Autodesk Inventor part; units mm, degrees
ref_plane "YZ Plane" through (0, 0, 0) normal (1, 0, 0) x (0, 1, 0)
ref_plane "XZ Plane" through (0, 0, 0) normal (0, 1, 0) x (-1, 0, 0)
ref_plane "XY Plane" through (0, 0, 0) normal (0, 0, 1) x (1, 0, 0)
sketch "Boceto1" plane through (0, 0, 0) normal (0, 1, 0) x (-1, 0, 0)
  line L0 (-12.5, 6.5) -> (12.5, 6.5)
  line L1 (12.5, 6.5) -> (12.5, -6.5)
  line L2 (12.5, -6.5) -> (-12.5, -6.5)
  line L3 (-12.5, -6.5) -> (-12.5, 6.5)
  line L4 (-12.5, 6.5) -> (12.5, -6.5) construction
  line L5 (12.5, 6.5) -> (-12.5, -6.5) construction
  point P0 (0, 0)
  dimension "d0" = 13
  dimension "d1" = 25
extrude "Extrusión1" add sketch "Boceto1" along normal blind 1.5
sketch "Boceto2" plane through (0, 1.5, 0) normal (0, 1, 0) x (1, 0, 0)
  circle A0 centre (-3.5, 0) radius 2.75
  line L0 (-12.5, 6.5) -> (-12.5, -6.5)
  point P0 (0, 0)
  dimension "d4" = 9
  dimension "d5" = 5.5
extrude "Extrusión2" cut sketch "Boceto2" against normal blind 1.5
sketch "Boceto3" plane through (0, 1.5, 0) normal (0, 1, 0) x (1, 0, 0)
  line L0 (-9.2, -5.5) -> (2.8, -5.5)
  line L1 (2.8, -5.5) -> (2.8, 5.5)
  line L2 (2.8, 5.5) -> (-9.2, 5.5)
  line L3 (-9.2, 5.5) -> (-9.2, -5.5)
  line L4 (-12.5, 6.5) -> (-12.5, -6.5)
  line L5 (12.5, 6.5) -> (-12.5, 6.5)
  circle A0 centre (-3.5, 0) radius 2.75
  circle A1 centre (-3.5, 0) radius 2
  point P0 (0, 0)
  dimension "d8" = 11
  dimension "d9" = 12
  dimension "d10" = 3.3
  dimension "d11" = 1
  dimension "d14" = 4
extrude "Extrusión3" add sketch "Boceto3" along normal blind 2 contours L3 L2 L1 L0 | A0
chamfer "Chaflán1" distance 3 angle 45 2 edges at (-9.2, 2.5, 5.5) (-9.2, 2.5, -5.5)
sketch "Boceto4" plane through (0, 3.5, 0) normal (0, 1, 0) x (1, 0, 0)
  circle A0 centre (-3.5, 0) radius 2
  line L0 (-2.5075, -1.7363) -> (-2.5075, 1.7363)
  point P0 (0, 0)
extrude "Extrusión4" add sketch "Boceto4" against normal up to surface (2 mm away) contours A0 L0 picked at (-2.1717, 0)
properties part number "AngleSensor"
The listing builds one solid part. Answer for the finished solid, in the listing's coordinates (mm). A direction names the side the tool comes from. Coordinates: 2 decimals unless noted, no trailing zeros. Write each loop counter-clockwise with the first axis right and the second up, starting at its lowest first coordinate (ties: lowest second). Pieces come first, ordered by that corner, then holes. Notation, with made-up numbers: M 47.5,-37.75 L 84.5,-37.75 A16 cw 84.5,-17.75 Z; hole C 74,67.25 d6. An arc over 180 degrees is marked long. Use one line per item in the form item = value.
Item 1: Find section B-B, the plane z = 0. Give the vertices of the cut face in (x, y), plus the area to 3 significant figures.
Model answer:
outline = M -12.5,0 L -6.25,0 L -6.25,1.5 L -5.5,1.5 L -5.5,3.5 L -9.2,3.5 L -9.2,1.5 L -12.5,1.5 Z; M -2.51,1.5 L -0.75,1.5 L -0.75,0 L 12.5,0 L 12.5,1.5 L 2.8,1.5 L 2.8,3.5 L -2.51,3.5 Z
area = 47.3 mm2
Item 2: Find section C-C, the plane z = -3. Give the vertices of the cut face in (x, y).
Model answer:
outline = M -12.5,0 L 12.5,0 L 12.5,1.5 L 2.8,1.5 L 2.8,3.5 L -8.7,3.5 L -8.7,1.5 L -12.5,1.5 Z
Item 3: Find section D-D, the plane x = 2.5. Give the vertices of the cut face in (y, z), plus the area to 3 significant figures.
Model answer:
outline = M 0,-6.5 L 1.5,-6.5 L 1.5,-5.5 L 3.5,-5.5 L 3.5,5.5 L 1.5,5.5 L 1.5,6.5 L 0,6.5 Z
area = 41.5 mm2
Item 4: The mould has two halves that part along Z. Classify faces 4 (the face through (3, 1.5, 0)), 5 (the face through (0, 1, -6.5)), 6 (the face through (-2, 2, 5.5)), 7 (the face through (-0.96, 0.76, 1.05)): released by +Z, released by -Z, zero draft, split by the parting line, or undercut.
Model answer:
face_4 = zero draft
face_5 = released by -Z
face_6 = released by +Z
face_7 = undercut
Item 5: Find section A-A, the plane x = -3.5. Give the vertices of the cut face in (y, z).
Model answer:
outline = M 0,-6.5 L 1.5,-6.5 L 1.5,-5.5 L 3.5,-5.5 L 3.5,-2 L 1.5,-2 L 1.5,-2.75 L 0,-2.75 Z; M 0,2.75 L 1.5,2.75 L 1.5,2 L 3.5,2 L 3.5,5.5 L 1.5,5.5 L 1.5,6.5 L 0,6.5 Z
Item 6: Find the intervals of material crossed by probe 1 along Z at (x, y) = (-3.5, 3.05); probe 2 along X at (y, z) = (0.35, 0); probe 3 along Z at (x, y) = (-3.5, 0.45), in increasing order.
Model answer:
probe_1 = -5.5 to -2, 2 to 5.5
probe_2 = -12.5 to -6.25, -0.75 to 12.5
probe_3 = -6.5 to -2.75, 2.75 to 6.5
Item 7: For faces 1 (the face through (-9.2, 2, 0)), 2 (the face through (-2.508, 3, 0)), 3 (the face through (-7.7, 2.5, -4)), determine the directions among +Z, -Z, +X, -X, +Y, -Y from which every point of the face is accessible in a straight line to the end or side of a thin tool.
Model answer:
face_1 = +Z, -Z, -X, +Y
face_2 = +Y, -Y
face_3 = -Z, -X, +Y
Item 8: Given P1, Ø1, axis at x = -2.5, y = 3, coming from the +Z side; P2, Ø0.6, axis at y = 3, z = 0.5, coming from the -X side; P3, Ø1.6, axis at x = -1, y = 3, coming from the -Z side, each flat-ended and moving along its own axis, determine where each tip first touches the part or whether it passes through.
Model answer:
P1 = 5.5
P2 = -9.2
P3 = -5.5
